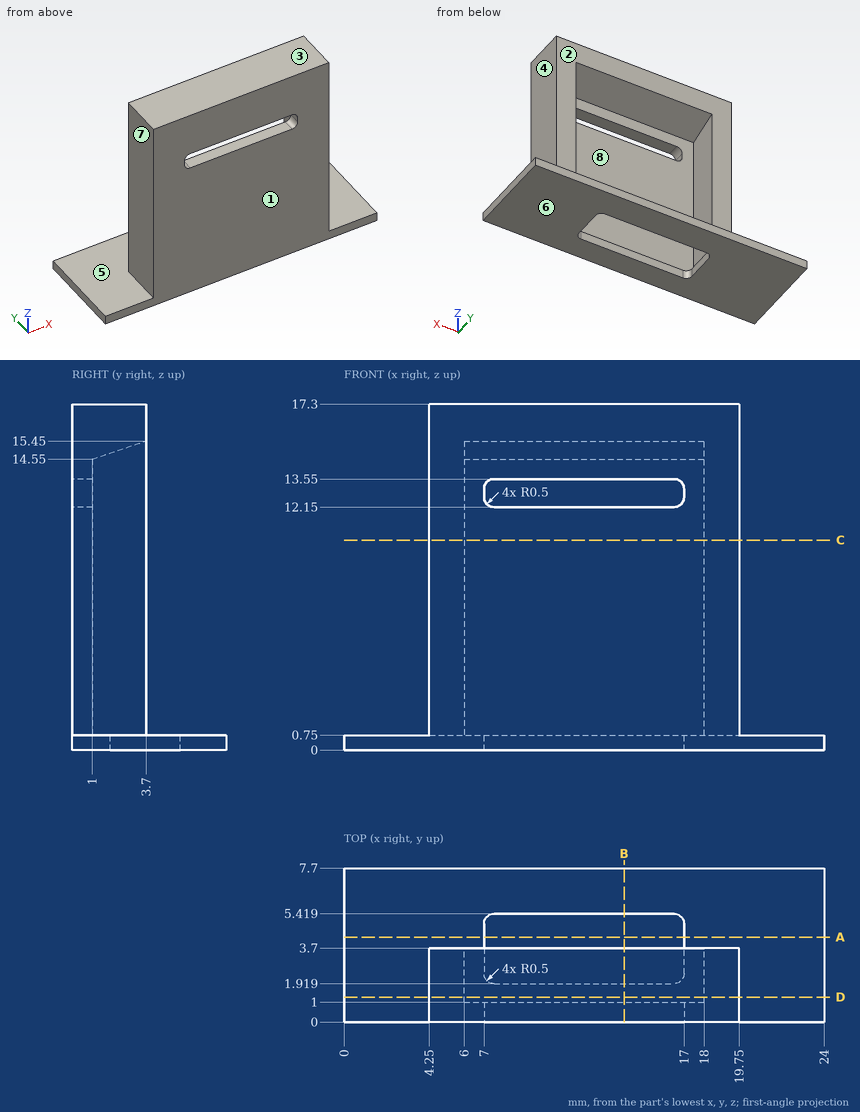
Source: three-view drawing plus pictorial views. Frame: mm from the lowest corner of the part. A direction names the side the tool comes from. Give positions to 0.01 mm unless a question says otherwise; leave off trailing zeros. Loops run counter-clockwise (first coordinate to the right, second up) from the corner with the lowest first, then second, coordinate; pieces in that order, holes last. Notation, with made-up numbers: (41, 80) -> (57, 80) arc R26 ccw to (57, 116) -> close; hole circle Ø9 at (5.5, 49). An arc over 180 degrees is marked (long way). Put each result on its own line as item: value. Start each with the question number.
1) Contact query for flat-ended pins moving along their axis: P1, Ø3, axis at y = 3, z = 4.5, coming from the +X side; P2, Ø5, axis at x = 9.5, z = 14, coming from the +Y side; P3, Ø1, axis at y = 4, z = 8.5, coming from the -X side. Output: stop coordinate, or through.
2) Cut plane A-A (y = 4.25). Return loops of the section in (x, z).
3) Cut plane B-B (x = 14). Return loops of the section in (y, z).
4) Draft query along X for the marked faces 6, 7 and 8. Return one class per face: released by +X, released by -X, zero draft, split by the parting line, or undercut.
5) Cut plane D-D (y = 1.25). Return loops of the section in (x, z).
6) Cut plane C-C (z = 10.5). Return loops of the section in (x, y).
7) Material intervals for probe 1 along X at (y, z) = (2.5, 12.75); probe 2 along X at (y, z) = (0.5, 9.5); probe 3 along Y at (x, z) = (9.25, 8), sorted ascending.
8) Reachability of the marked faces 1, 2, 3, 4 and 5 from +Z, -Z, +X, -X, +Y, -Y: full face, straight path, thin tool, end or side. Return the list, or none.
Results are:
1. P1: stops at x = 19.75
1. P2: stops at y = 3.7
1. P3: stops at x = 4.25
2. outline: (0, 0) -> (7, 0) -> (7, 0.75) -> (0, 0.75) -> close; (17, 0) -> (24, 0) -> (24, 0.75) -> (17, 0.75) -> close
3. outline: (0, 0) -> (1.92, 0) -> (1.92, 0.75) -> (1, 0.75) -> (1, 12.15) -> (0, 12.15) -> close; (0, 13.55) -> (1, 13.55) -> (1, 14.55) -> (3.7, 15.45) -> (3.7, 17.3) -> (0, 17.3) -> close; (5.42, 0) -> (7.7, 0) -> (7.7, 0.75) -> (5.42, 0.75) -> close
4. face 6: zero draft
4. face 7: released by -X
4. face 8: undercut
5. outline: (0, 0) -> (24, 0) -> (24, 0.75) -> (19.75, 0.75) -> (19.75, 17.3) -> (4.25, 17.3) -> (4.25, 0.75) -> (0, 0.75) -> close; hole (6, 0.75) -> (18, 0.75) -> (18, 14.63) -> (6, 14.63) -> close
6. outline: (4.25, 0) -> (19.75, 0) -> (19.75, 3.7) -> (18, 3.7) -> (18, 1) -> (6, 1) -> (6, 3.7) -> (4.25, 3.7) -> close
7. probe 1: x = 4.25 to 6, 18 to 19.75
7. probe 2: x = 4.25 to 19.75
7. probe 3: y = 0 to 1
8. face 1: +Z, -Z, +X, -X, -Y
8. face 2: +Z, +X, -X, +Y
8. face 3: +Z, +X, -X, +Y, -Y
8. face 4: +Z, +X, +Y, -Y
8. face 5: +Y
